Work out the finished part from the listing and answer in its coordinate system (mm). A direction names the side the tool comes from. Coordinates: 2 decimals unless noted, no trailing zeros. Order: outer loops, then holes, each group sorted by start corner. A loop starts at its lowest first (then second) coordinate and runs counter-clockwise, first axis right, second up. Notation, with made-up numbers: M 68.5,76 L 108.5,76 A20 cw 108.5,80 Z; hole C 49.5,-14 d3. An arc over 180 degrees is marked long. Answer in a Markdown table with one row per item. Add a question column.
Item 1: The part is cut by section A-A (z = 0). Write down the section's boundary in (x, y).
Item 2: The part is cut by section B-B (x = -6.75). Write down the section's boundary in (y, z).
Item 3: Which of the six approach directions +Z, -Z, +X, -X, +Y, -Y give full straight-line access (tool end or side, diameter ignored) to faces 1 (the face through (-5.8, 4.7, 0)), 2 (the face through (5.8, 4.7, 0)), 3 (the face through (-1.78, 4.7, -5.52)), 4 (the face through (0, 4.7, 5.8))?
Item 4: The part is cut by section C-C (y = 0.75). Write down the section's boundary in (x, z), then the cut area to 3 significant figures.
Item 5: The mould has two halves that part along Z. Classify faces 5 (the face through (5.513, 4.698, 1.802)), 6 (the face through (-1.172, 8.993, 8.923)), 7 (the face through (0, 4.7, -5.8)): released by +Z, released by -Z, zero draft, split by the parting line, or undercut.
Item 6: Consider line 1 (X direction, y = 7, z = 0); line 2 (Y direction, x = 0.5, z = 7.5). Determine where each line is inside the solid, lowest interval first. Write a range as from..to.
Item 7: The part is cut by section D-D (x = 0). Write down the section's boundary in (y, z).
Item 8: Flat-ended cylindrical pins translate along their axes: pin 1 Ø1.5 at (y, z) = (3.5, 7) entering from +X; pin 2 Ø1 at (x, y) = (0, 7.5) entering from -Z. Find the tip coordinate at first contact, or state that the pin passes through.
Autodesk Inventor part; units mm, degrees
ref_plane "YZ Plane" through (0, 0, 0) normal (1, 0, 0) x (0, 1, 0)
ref_plane "XZ Plane" through (0, 0, 0) normal (0, 1, 0) x (-1, 0, 0)
ref_plane "XY Plane" through (0, 0, 0) normal (0, 0, 1) x (1, 0, 0)
sketch "Sketch1" plane through (0, 0, 0) normal (0, 0, 1) x (1, 0, 0)
  line L0 (0, 0) -> (0, 9.5) construction
  line L1 (0, 9.5) -> (2.5, 9.5) construction
  line L2 (2.5, 9.5) -> (9, 9.5)
  line L3 (9, 9.5) -> (9, 8.5)
  line L4 (9, 8.5) -> (6.1, 8.5)
  line L5 (6.1, 8.5) -> (6.1, 1)
  line L6 (6.1, 1) -> (9, 1)
  line L7 (9, 1) -> (9, 0)
  line L8 (9, 0) -> (2.5, 0)
  line L9 (2.5, 0) -> (2.5, 9.5)
  dimension "d0" = 2.5
  dimension "d1" = 7.5
  dimension "d2" = 1
  dimension "d3" = 9
  dimension "d4" = 1
  dimension "d6" = 6.1
revolve "Revolution1" add sketch "Sketch1" angle 360 about axis through (0, 0, 0) along (0, 1, 0)
sketch "Sketch2" plane through (0, 1, 0) normal (0, 1, 0) x (1, 0, 0)
  line L0 (0, 0) -> (6.8, 0)
  circle A0 centre (6.8, 0) radius 1
  dimension "d8" = 6.8
  dimension "d9" = 2
extrude "Extrusion1" cut sketch "Sketch2" along normal up to surface (7.5 mm away)
pattern_circular "Circular Pattern1" count 20 over 360 about axis through (0, 4.75, 0) along (0, -1, 0) of "Extrusion1"
properties part number "20t GT2 Idler"
Reply:
| question | item | result |
|---|---|---|
| 1 | outline | M -9,0 L -2.5,0 L -2.5,9.5 L -9,9.5 L -9,8.5 L -5.8,8.5 L -5.8,1 L -9,1 Z; M 2.5,0 L 9,0 L 9,1 L 5.8,1 L 5.8,8.5 L 9,8.5 L 9,9.5 L 2.5,9.5 Z |
| 2 | outline | M 0,-5.95 L 1,-5.95 L 1,5.95 L 0,5.95 Z; M 8.5,-5.95 L 9.5,-5.95 L 9.5,5.95 L 8.5,5.95 Z |
| 3 | face 1 | -X |
| 3 | face 2 | +X |
| 3 | face 3 | -Z |
| 3 | face 4 | +Z |
| 4 | outline | C 0,0 d18; hole C 0,0 d5 |
| 4 | area | 235 mm2 |
| 5 | face 5 | undercut |
| 5 | face 6 | split by the parting line |
| 5 | face 7 | released by -Z |
| 6 | line 1 | x = -5.8..-2.5, 2.5..5.8 |
| 6 | line 2 | y = 0..1, 8.5..9.5 |
| 7 | outline | M 0,-9 L 1,-9 L 1,-5.8 L 8.5,-5.8 L 8.5,-9 L 9.5,-9 L 9.5,-2.5 L 0,-2.5 Z; M 0,2.5 L 9.5,2.5 L 9.5,9 L 8.5,9 L 8.5,5.8 L 1,5.8 L 1,9 L 0,9 Z |
| 8 | pin 1 | passes through |
| 8 | pin 2 | stops at z = -5.93 |
